Source: CAD feature listing. Evaluate the final solid. Frame: model axes, mm. Face numbers are marked on the shaded views. A direction names the side the tool comes from. Coordinates: 2 decimals unless noted, no trailing zeros. Loops run counter-clockwise (first coordinate to the right, second up) from the corner with the lowest first, then second, coordinate; pieces in that order, holes last. Notation, with made-up numbers: (67.5, 89) -> (84.5, 89) arc R19 cw to (84.5, 95) -> close; hole circle Ø2 at (44.5, -4.5). An arc over 180 degrees is marked (long way). Answer as a JSON object with one key per item and string values. Group by question number.
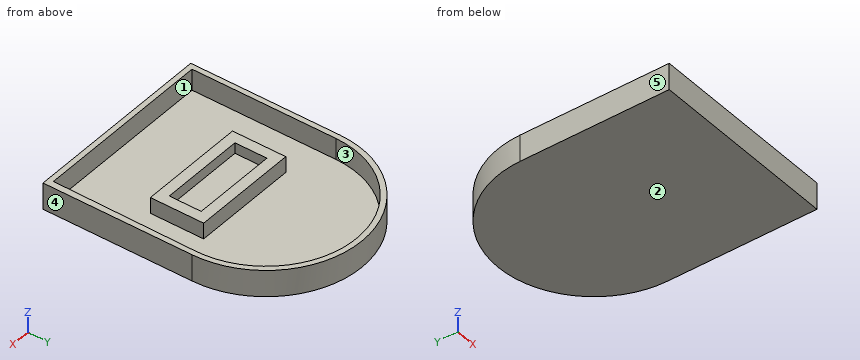
from build123d import *

# Parameters (mm, degrees)
BOSS_EXTRUDE1_DEPTH = 20
BOSS_EXTRUDE2_START = 5
BOSS_EXTRUDE2_DEPTH = 5
SKETCH3_W           = 100
SKETCH3_H           = 50
BOSS_EXTRUDE3_DEPTH = 15
SHELL1_T            = -10


with BuildPart() as part:
    # Sketch1 → Boss-Extrude1 (new body)
    with BuildSketch(Plane.XY):
        with BuildLine():
            Line((-90, 0), (-90, -140))
            Line((-90, -140), (90, -140))
            Line((90, -140), (90, 0))
            ThreePointArc((90, 0), (0, 90), (-90, 0))
        make_face()
        with BuildLine():
            Line((-85, 0), (-85, -135))
            Line((-85, -135), (83.811538659, -135))
            Line((83.811538659, -135), (84.986825994, -1.496464972))
            ThreePointArc((84.986825994, -1.496464972), (0.74826148, 84.996706435), (-85, 0))
        make_face(mode=Mode.SUBTRACT)
    extrude(amount=BOSS_EXTRUDE1_DEPTH)

    # Sketch2 → Boss-Extrude2 (add)
    with BuildSketch(Plane(origin=(0, 0, 0), x_dir=(-1, 0, 0), z_dir=(0, 0, -1)).offset(BOSS_EXTRUDE2_START)):
        with BuildLine():
            Line((-90, 0), (-90, -140))
            Line((-90, -140), (90, -140))
            Line((90, -140), (90, 0))
            ThreePointArc((90, 0), (0, 90), (-90, 0))
        make_face()
    extrude(amount=-BOSS_EXTRUDE2_DEPTH)

    # Sketch3 → Boss-Extrude3 (add)
    with BuildSketch(Plane.XY):
        with Locations((0, -45)):
            Rectangle(SKETCH3_W, SKETCH3_H)
    extrude(amount=BOSS_EXTRUDE3_DEPTH)

    # Shell1
    shell1_openings = [part.faces().sort_by_distance(p)[0] for p in [
        (0, -45, 15),
    ]]
    offset(amount=SHELL1_T, openings=shell1_openings)


solid = part.part
1. Section query A-A on z = 9. Return loops of the section in (x, y).
2. Section query D-D on y = 8. Return loops of the section in (x, z).
3. Ray query, L1, parallel to Y at x = 41, z = 2.5; L2, parallel to Y at x = 33.5, z = 9.5; L3, parallel to Y at x = 33, z = 13.5. Return the intervals inside material, ascending.
4. Reachability of the marked faces 1 and 2 from +Z, -Z, +X, -X, +Y, -Y: full face, straight path, thin tool, end or side. Return the list, or none.
5. Section query C-C on y = -73. Return loops of the section in (x, z).
6. Pin query (flat end, axial travel): pin 1 Ø9 at (x, y) = (-10.5, -50) entering from +Z; pin 2 Ø15 at (x, y) = (-9, -37) entering from +Z; pin 3 Ø12 at (y, z) = (61.5, -2) entering from +X. Return the tip coordinate at first contact, or that it passes through.
7. Section query B-B on x = 0. Return loops of the section in (y, z).
8. Mould query, pull axis X, two halves, no side actions, for the marked faces 3, 4 and 5. Classes: pulls with the +X half, pulls with the -X half, needs draft (parallel to the pull), parting line crosses it, or undercut.
Solved:
{
 "1": {"outline": "(-90, -140) -> (90, -140) -> (90, 0) arc R90 ccw to (-90, 0) -> close; (-50, -70) -> (50, -70) -> (50, -20) -> (-50, -20) -> close; hole (-85, -135) -> (83.81, -135) -> (84.99, -1.5) arc R85 ccw (long way) to (-85, 0) -> close; hole (-40, -60) -> (40, -60) -> (40, -30) -> (-40, -30) -> close"},
 "2": {"outline": "(-89.64, -5) -> (89.64, -5) -> (89.64, 20) -> (84.62, 20) -> (84.62, 0) -> (-84.62, 0) -> (-84.62, 20) -> (-89.64, 20) -> close"},
 "3": {"L1": "-140 to -135, -70 to -20, 74.46 to 80.12", "L2": "-140 to -135, -70 to -60, -30 to -20, 78.12 to 83.53", "L3": "-140 to -135, -70 to -60, -30 to -20, 78.33 to 83.73"},
 "4": {"face 1": "+Z", "face 2": "-Z, +X, -X, +Y, -Y"},
 "5": {"outline": "(-90, -5) -> (90, -5) -> (90, 20) -> (84.36, 20) -> (84.36, 0) -> (-85, 0) -> (-85, 20) -> (-90, 20) -> close"},
 "6": {"pin 1": "z = 5", "pin 2": "z = 15", "pin 3": "x = 70.85"},
 "7": {"outline": "(-140, -5) -> (90, -5) -> (90, 20) -> (85, 20) -> (85, 0) -> (-20, 0) -> (-20, 15) -> (-30, 15) -> (-30, 5) -> (-60, 5) -> (-60, 15) -> (-70, 15) -> (-70, 0) -> (-135, 0) -> (-135, 20) -> (-140, 20) -> close"},
 "8": {"face 3": "undercut", "face 4": "pulls with the +X half", "face 5": "pulls with the -X half"}
}
